Build history of the part. All positions in model axes, mm. Face numbers are marked on the shaded views. A direction names the side the tool comes from. Round coordinates to 2 decimals unless told otherwise and drop trailing zeros. Loops run counter-clockwise (first coordinate to the right, second up) from the corner with the lowest first, then second, coordinate; pieces in that order, holes last. Notation, with made-up numbers: (-15.75, 61.25) -> (33.25, 61.25) arc R30 cw to (33.25, 91.25) -> close; hole circle Ø10 at (89.5, 36.5). An arc over 180 degrees is marked (long way). Put each result on its own line as item: value. Start each with the question number.
Item 1: Flat gauge pins, fed straight in: pin 1 Ø4.5 at (x, y) = (0, 0) entering from +Z; pin 2 Ø1 at (x, z) = (1, 14) entering from +Y; pin 3 Ø1 at (x, z) = (-3.5, 12) entering from +Y. Where does each tip first touch, or does it go through?
Item 2: Cut at A-A, the plane y = 0. List the corners of the cut face in (x, z).
Item 3: Pull direction Y, two halves, no side cores. Call the marked faces 1, 2, 3 and 4: +Y half, -Y half, draft (parallel to the pull), parting line (faces both ways), or undercut.
Item 4: Cut at B-B, the plane x = 6.25. List the corners of the cut face in (y, z).
Item 5: Drill centre lines: probe 1 along Y at (x, z) = (0, 10); probe 2 along Y at (x, z) = (-12, 3.75); probe 3 along Z at (x, y) = (6.25, 5). Where is each one in solid material? Low to high. Write a range as [from, to].
Item 6: Tool access for the marked faces 5 and 6: list every direction of +Z, -Z, +X, -X, +Y, -Y with a clear straight run to the whole face (end or side of a thin tool).
Item 7: Cut at C-C, the plane z = 12. List the corners of the cut face in (x, y), plus the area to 3 significant figures.
```python
from build123d import *

# Parameters (mm, degrees)
SKETCH_1_W          = 30
SKETCH_1_H          = 30
EXTRUDE_1_DEPTH     = 4
FILLET_1_R          = 2
SHELL_1_T           = -1
SKETCH_2_R          = 3.4
EXTRUDE_2_DEPTH     = 15
SKETCH_3_R          = 2.9
CUT_EXTRUDE_1_DEPTH = 15


with BuildPart() as part:
    # 草图1 → 凸台-拉伸1 (new body)
    with BuildSketch(Plane.XY):
        Rectangle(SKETCH_1_W, SKETCH_1_H)
    extrude(amount=EXTRUDE_1_DEPTH)

    # 圆角1
    fillet_1_edges = [part.edges().sort_by_distance(p)[0] for p in [
        (0, -15, 0),
        (-15, 0, 0),
        (0, 15, 0),
        (15, 0, 0),
        (15, -15, 2),
        (-15, -15, 2),
        (-15, 15, 2),
        (15, 15, 2),
    ]]
    fillet(fillet_1_edges, radius=FILLET_1_R)

    # 抽壳1
    shell_1_openings = [part.faces().sort_by_distance(p)[0] for p in [
        (0, 0, 4),
    ]]
    offset(amount=SHELL_1_T, openings=shell_1_openings, kind=Kind.INTERSECTION)

    # 草图2 → 凸台-拉伸2 (add)
    with BuildSketch(Plane.XY.offset(1)):
        Circle(SKETCH_2_R)
    extrude(amount=EXTRUDE_2_DEPTH)

    # 草图3 → 切除-拉伸1 (cut)
    with BuildSketch(Plane.XY.offset(16)):
        Circle(SKETCH_3_R)
    extrude(amount=-CUT_EXTRUDE_1_DEPTH, mode=Mode.SUBTRACT)


solid = part.part
```
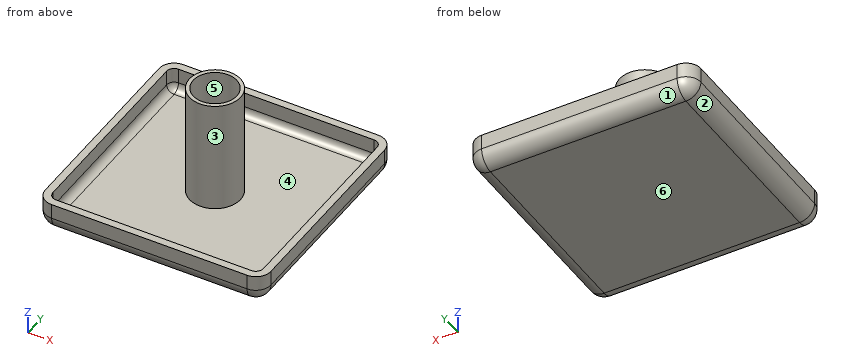
Reply:
1. pin 1: stops at z = 1
1. pin 2: stops at y = 3.36
1. pin 3: stops at y = 1.6
2. outline: (-15, 2) arc R2 ccw to (-13, 0) -> (13, 0) arc R2 ccw to (15, 2) -> (15, 4) -> (14, 4) -> (14, 2) arc R1 cw to (13, 1) -> (3.4, 1) -> (3.4, 16) -> (2.9, 16) -> (2.9, 1) -> (-2.9, 1) -> (-2.9, 16) -> (-3.4, 16) -> (-3.4, 1) -> (-13, 1) arc R1 cw to (-14, 2) -> (-14, 4) -> (-15, 4) -> close
3. face 1: +Y half
3. face 2: draft
3. face 3: undercut
3. face 4: undercut
4. outline: (-15, 2) arc R2 ccw to (-13, 0) -> (13, 0) arc R2 ccw to (15, 2) -> (15, 4) -> (14, 4) -> (14, 2) arc R1 cw to (13, 1) -> (-13, 1) arc R1 cw to (-14, 2) -> (-14, 4) -> (-15, 4) -> close
5. probe 1: y = [-3.4, -2.9], [2.9, 3.4]
5. probe 2: y = [-15, -14], [14, 15]
5. probe 3: z = [0, 1]
6. face 5: +Z
6. face 6: -Z, +X, -X, +Y, -Y
7. outline: circle Ø6.8 at (0, 0); hole circle Ø5.8 at (0, 0)
7. area: 9.90 mm^2
